Build history of the part. All positions in model axes, mm. Face numbers are marked on the shaded views. A direction names the side the tool comes from. Give positions to 0.01 mm unless a question says otherwise; leave off trailing zeros. Loops run counter-clockwise (first coordinate to the right, second up) from the corner with the lowest first, then second, coordinate; pieces in that order, holes last. Notation, with made-up numbers: (-22.5, 16.25) -> (23.5, 16.25) arc R14 cw to (23.5, 43.25) -> close; hole circle Ø2 at (67, 83.5). An arc over 180 degrees is marked (long way). Answer as a JSON object with one key per item and string values. Group by question number.
Q1. Tool access for the marked faces 4, 5 and 6: list every direction of +Z, -Z, +X, -X, +Y, -Y with a clear straight run to the whole face (end or side of a thin tool).
Q2. Band-saw the part on D-D, the plane x = -13.5. Write the cut outline in (y, z), plus the area to 3 significant figures.
Q3. Wall check: probe 1 along Y at (x, z) = (0, 8); probe 2 along Z at (x, y) = (-1.5, 18.5); probe 3 along Y at (x, z) = (18, 26). Give the ranges that are in metal, low to high. Write a range as from..to.
Q4. Band-saw the part on B-B, the plane z = 6. Write the cut outline in (x, y).
Q5. Drop flat-ended pins along their axis: pin 1 (8 mm diameter, centred on x = -3.5, z = 38.5, fed in from +Y); pin 2 (1 mm diameter, centred on y = 29, z = 13.5, fed in from +X); pin 3 (23 mm diameter, centred on x = 0, y = 33, fed in from +Z). Give the stop position or say it passes through.
Q6. Band-saw the part on A-A, the plane x = 0. Write the cut outline in (y, z).
Q7. Two-plate mould, pull along Y, no slides. Class the marked faces 1, 2 and 3: pulls with the +Y half, pulls with the -Y half, needs draft (parallel to the pull), parting line crosses it, or undercut.
Q8. Band-saw the part on C-C, the plane y = 33. Write the cut outline in (x, z), plus the area to 3 significant figures.
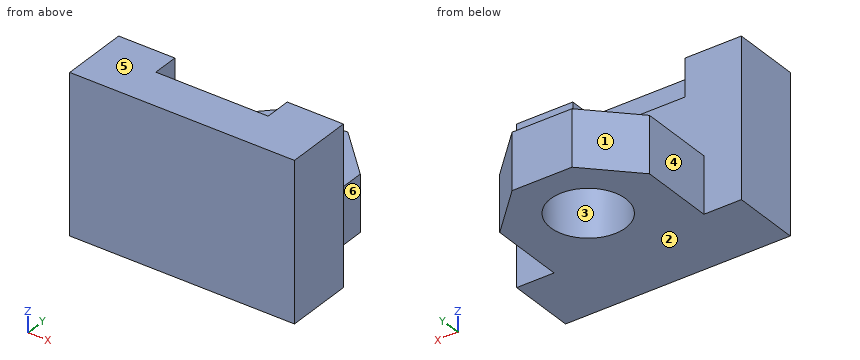
from build123d import *

# Parameters (mm, degrees)
SKETCH1_W           = 60
SKETCH1_H           = 18
BOSS_EXTRUDE1_DEPTH = 42
SKETCH2_W           = 30
SKETCH2_H           = 10
CUT_EXTRUDE1_DEPTH  = 7
BOSS_EXTRUDE2_DEPTH = 15
SKETCH4_R           = 10
CUT_EXTRUDE2_DEPTH  = 65.257295306


with BuildPart() as part:
    # Sketch1 → Boss-Extrude1 (new body)
    with BuildSketch(Plane.XY):
        with Locations((0, 9)):
            Rectangle(SKETCH1_W, SKETCH1_H)
    extrude(amount=BOSS_EXTRUDE1_DEPTH)

    # Sketch2 → Cut-Extrude1 (cut)
    with BuildSketch(Plane(origin=(0, 18, 0), x_dir=(1, 0, 0), z_dir=(0, 1, 0))):
        with Locations((0, -37)):
            Rectangle(SKETCH2_W, SKETCH2_H)
    extrude(amount=-CUT_EXTRUDE1_DEPTH, mode=Mode.SUBTRACT)

    # Sketch3 → Boss-Extrude2 (add)
    with BuildSketch(Plane(origin=(0, 0, 0), x_dir=(-1, 0, 0), z_dir=(0, 0, -1))):
        Polygon((20, 18), (20, 38), (8, 50), (-8, 50), (-20, 38), (-20, 18), align=None)
    extrude(amount=-BOSS_EXTRUDE2_DEPTH)

    # Sketch4 → Cut-Extrude2 (cut, through all)
    with BuildSketch(Plane.XY.offset(15)):
        with Locations((0, 33)):
            Circle(SKETCH4_R)
    extrude(amount=-CUT_EXTRUDE2_DEPTH, mode=Mode.SUBTRACT)


solid = part.part
Worked answers:
{
 "1": {"face 4": "+Z, -Z, -X, +Y", "face 5": "+Z, +X, -X, +Y, -Y", "face 6": "+Z, -Z, +X, +Y"},
 "2": {"outline": "(0, 0) -> (44.5, 0) -> (44.5, 15) -> (18, 15) -> (18, 32) -> (11, 32) -> (11, 42) -> (0, 42) -> close", "area": "1,080 mm2"},
 "3": {"probe 1": "0..23, 43..50", "probe 2": "0..15", "probe 3": "0..18"},
 "4": {"outline": "(-30, 0) -> (30, 0) -> (30, 18) -> (20, 18) -> (20, 38) -> (8, 50) -> (-8, 50) -> (-20, 38) -> (-20, 18) -> (-30, 18) -> close; hole circle Ø20 at (0, 33)"},
 "5": {"pin 1": "y = 11", "pin 2": "x = 20", "pin 3": "z = 15"},
 "6": {"outline": "(0, 0) -> (23, 0) -> (23, 15) -> (18, 15) -> (18, 32) -> (11, 32) -> (11, 42) -> (0, 42) -> close; (43, 0) -> (50, 0) -> (50, 15) -> (43, 15) -> close"},
 "7": {"face 1": "pulls with the +Y half", "face 2": "needs draft", "face 3": "undercut"},
 "8": {"outline": "(-20, 0) -> (-10, 0) -> (-10, 15) -> (-20, 15) -> close; (10, 0) -> (20, 0) -> (20, 15) -> (10, 15) -> close", "area": "300 mm2"}
}
